from build123d import *

# Parameters (mm, degrees)
BOSS_EXTRUDE1_DEPTH = 170


with BuildPart() as part:
    # Sketch1 → Boss-Extrude1 (new body, symmetric)
    with BuildSketch(Plane.XY):
        Polygon((-2.585786438, 4), (2.585786438, 4), (6.585786438, 8), (2.5, 8), (2.5, 10), (10, 10), (10, 2.5), (8, 2.5), (8, 6.585786438), (4, 2.585786438), (4, -2.585786438), (8, -6.585786438), (8, -2.5), (10, -2.5), (10, -10), (2.5, -10), (2.5, -8), (6.585786438, -8), (2.585786438, -4), (-2.585786438, -4), (-6.585786438, -8), (-2.5, -8), (-2.5, -10), (-10, -10), (-10, -2.5), (-8, -2.5), (-8, -6.585786438), (-4, -2.585786438), (-4, 2.585786438), (-8, 6.585786438), (-8, 2.5), (-10, 2.5), (-10, 10), (-2.5, 10), (-2.5, 8), (-6.585786438, 8), align=None)
    extrude(amount=BOSS_EXTRUDE1_DEPTH, both=True)


solid = part.part
Read the model definition and answer for the solid it produces. Units are mm, in the model's axes. Round coordinates to 2 decimals unless told otherwise and drop trailing zeros.
1. Given pin 1 Ø1.5 at (x, y) = (5.5, -2) entering from -Z; pin 2 Ø4 at (x, z) = (0, -43.5) entering from +Y; pin 3 Ø3 at (y, z) = (-0.5, 81.5) entering from +X; pin 4 Ø1.6 at (x, z) = (-0.5, -70) entering from -Y, each flat-ended and moving along its own axis, determine where each tip first touches the part or whether it passes through.
2. Straight lines are drawn through the part: L1, parallel to X at y = -5, z = -98; L2, parallel to X at y = 3.25, z = -114; L3, parallel to Y at x = 8.75, z = -89.5. For each, find the intervals that lie inside material, in ascending order.
3. Determine the mould class of faces 1 (the face through (-4, 0, 2)), 2 (the face through (0, 0, -170)), 3 (the face through (-6, -10, 2)) for opening direction Y: pulls with the +Y half, pulls with the -Y half, needs draft (parallel to the pull), parting line crosses it, or undercut.
Values:
1. pin 1: passes through
1. pin 2: stops at y = 4
1. pin 3: stops at x = 4
1. pin 4: stops at y = -4
2. L1: x = -10 to -8, -6.41 to -3.59, 3.59 to 6.41, 8 to 10
2. L2: x = -10 to -8, -4.66 to 4.66, 8 to 10
2. L3: y = -10 to -2.5, 2.5 to 10
3. face 1: undercut
3. face 2: needs draft
3. face 3: pulls with the -Y half
